Answer from the drawing. Dimensions are ordinates in mm from the lowest x, y and z of the part. A direction names the side the tool comes from. Round coordinates to 2 decimals unless told otherwise and drop trailing zeros. Loops run counter-clockwise (first coordinate to the right, second up) from the corner with the lowest first, then second, coordinate; pieces in that order, holes last. Notation, with made-up numbers: (54, 13) - (79, 13) arc R22 ccw to (79, 42) - close; hole circle Ø8 at (27.5, -39). An arc over 180 degrees is marked (long way). One line per question, with ' | ' between items. Start each with the question number.
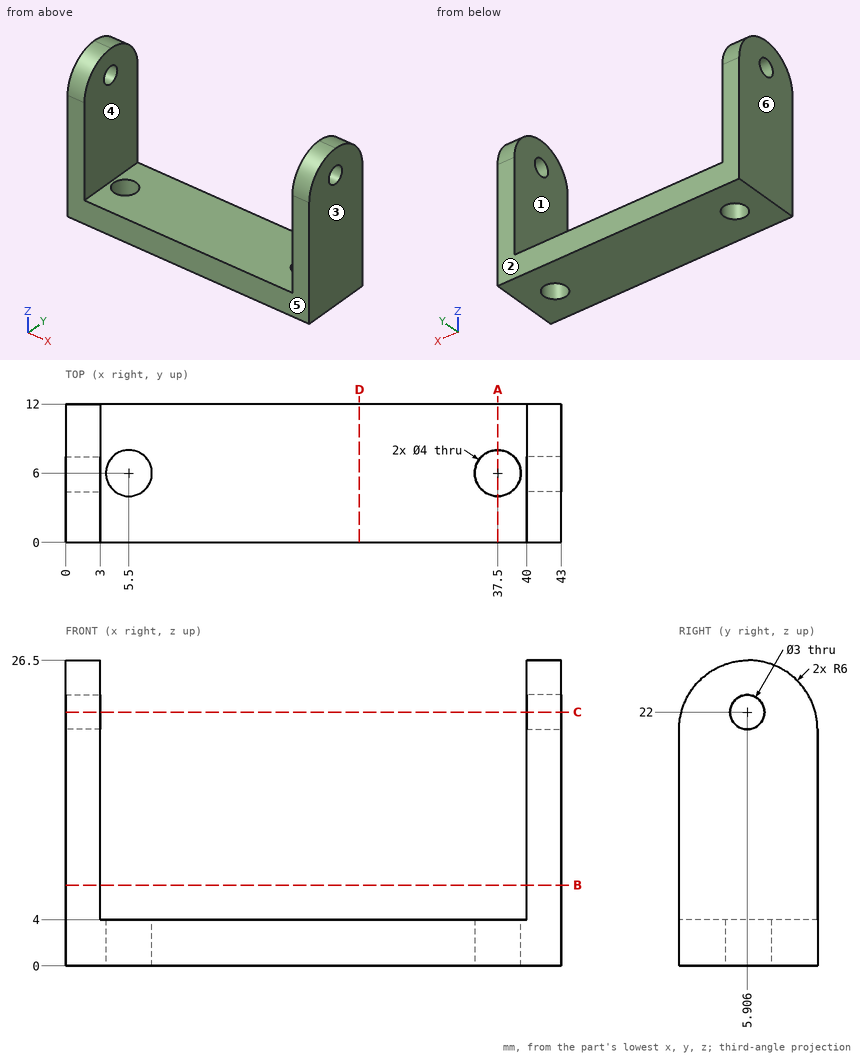
(1) Find section C-C on z = 22. Write down the section's boundary in (x, y), plus the area to 3 significant figures.
(2) Each of these flat-tipped pins is pushed along its axis until it touches: P1, Ø1.5, axis at x = 31.5, y = 9, coming from the +Z side; P2, Ø1.5, axis at y = 5.5, z = 22.5, coming from the +X side (3 decimals); P3, Ø1.5, axis at x = 33.5, y = 3.5, coming from the -Z side. Where does it stop, or does it pass through?
(3) Find section A-A on x = 37.5. Write down the section's boundary in (y, z).
(4) Determine the mould class of the marked faces 3, 4, 5 and 6 for opening direction X: pulls with the +X half, pulls with the -X half, needs draft (parallel to the pull), parting line crosses it, or undercut.
(5) Consider L1, parallel to X at y = 8.5, z = 6.5; L2, parallel to Z at x = 39.5, y = 8.5; L3, parallel to Y at x = 41.85, z = 22 (1 decimal). Determine where each line is inside the solid, lowest interval first.
(6) A tool of negligible diameter and unlimited length cuts with its end or side. For the marked faces 1 and 2, from which of +Z, -Z, +X, -X, +Y, -Y can it reach the whole face along a straight path? Write none if from no direction.
(7) Find section D-D on x = 25.5. Write down the section's boundary in (y, z), plus the area to 3 significant figures.
(8) Find section B-B on z = 7. Write down the section's boundary in (x, y), plus the area to 3 significant figures.
Answer below:
1) outline: (0, 0.19) - (3, 0.19) - (3, 4.41) - (0, 4.41) - close; (0, 7.41) - (3, 7.41) - (3, 11.81) - (0, 11.81) - close; (40, 0.19) - (43, 0.19) - (43, 4.41) - (40, 4.41) - close; (40, 7.41) - (43, 7.41) - (43, 11.81) - (40, 11.81) - close | area: 51.7 mm2
2) P1: z = 4 | P2: through | P3: z = 0
3) outline: (0, 0) - (4, 0) - (4, 4) - (0, 4) - close; (8, 0) - (12, 0) - (12, 4) - (8, 4) - close
4) face 3: pulls with the +X half | face 4: undercut | face 5: needs draft | face 6: pulls with the -X half
5) L1: 0 to 3, 40 to 43 | L2: 0 to 4 | L3: 0.2 to 4.4, 7.4 to 11.8
6) face 1: +Z, +Y, -Y | face 2: +Z, -Z, +X, -X, +Y
7) outline: (0, 0) - (12, 0) - (12, 4) - (0, 4) - close | area: 48.0 mm2
8) outline: (0, 0) - (3, 0) - (3, 12) - (0, 12) - close; (40, 0) - (43, 0) - (43, 12) - (40, 12) - close | area: 72.0 mm2
